```python
from build123d import *

# Parameters (mm, degrees)
SKETCH1_R           = 9.4
BOSS_EXTRUDE1_DEPTH = 13
SKETCH2_R           = 1
BOSS_EXTRUDE2_DEPTH = 5.75
SKETCH3_W           = 7.717079408
SKETCH3_H           = 3.649036098
SKETCH4_R           = 9.4
SKETCH4_R_2         = 0.762
CUT_EXTRUDE1_DEPTH  = 1.617316387


with BuildPart() as part:
    # Sketch1 → Boss-Extrude1 (new body)
    with BuildSketch(Plane.XY):
        with Locations(Location((0, 0, 0), (0, 0, 180))):
            Circle(SKETCH1_R)
    extrude(amount=BOSS_EXTRUDE1_DEPTH)

    # Sketch2 → Boss-Extrude2 (add)
    with BuildSketch(Plane.XY.offset(13)):
        Circle(SKETCH2_R)
    extrude(amount=BOSS_EXTRUDE2_DEPTH)

    # Sketch3 → Cut-Revolve1 (revolve, cut)
    with BuildSketch(Plane(origin=(0, 0, 0), x_dir=(1, 0, 0), z_dir=(0, 1, 0)), mode=Mode.PRIVATE) as cut_revolve1_sk:
        with Locations((5.541460296, -3.441834436)):
            Rectangle(SKETCH3_W, SKETCH3_H)
    revolve(cut_revolve1_sk.sketch.rotate(Axis((0, 0, 0), (0, 0, 1)), 180), axis=Axis((0, 0, 0), (0, 0, 1)), mode=Mode.SUBTRACT)

    # Sketch4 → Cut-Extrude1 (cut)
    with BuildSketch(Plane(origin=(0, 0, 0), x_dir=(-1, 0, 0), z_dir=(0, 0, -1))):
        Circle(SKETCH4_R)
        with BuildLine():
            ThreePointArc((-2.032, 5.588), (0, 7.62), (2.032, 5.588))
            ThreePointArc((2.032, 5.588), (3.073528286, 3.073528286), (5.588, 2.032))
            ThreePointArc((5.588, 2.032), (7.62, 0), (5.588, -2.032))
            ThreePointArc((5.588, -2.032), (3.073528286, -3.073528286), (2.032, -5.588))
            ThreePointArc((2.032, -5.588), (0, -7.62), (-2.032, -5.588))
            ThreePointArc((-2.032, -5.588), (-3.073528286, -3.073528286), (-5.588, -2.032))
            ThreePointArc((-5.588, -2.032), (-7.62, 0), (-5.588, 2.032))
            ThreePointArc((-5.588, 2.032), (-3.073528286, 3.073528286), (-2.032, 5.588))
        make_face(mode=Mode.SUBTRACT)
        with Locations((0, 5.588)):
            Circle(SKETCH4_R_2)
        with Locations((5.588, 0)):
            Circle(SKETCH4_R_2)
        with Locations((0, -5.588)):
            Circle(SKETCH4_R_2)
        with Locations((-5.588, 0)):
            Circle(SKETCH4_R_2)
    extrude(amount=-CUT_EXTRUDE1_DEPTH, mode=Mode.SUBTRACT)


solid = part.part
```
Build history of the part. All positions in model axes, mm. A direction names the side the tool comes from. Round coordinates to 2 decimals unless told otherwise and drop trailing zeros. Order: outer loops, then holes, each group sorted by start corner. A loop starts at its lowest first (then second) coordinate and runs counter-clockwise, first axis right, second up. Notation, with made-up numbers: (3, 6) - (56, 6) arc R8 cw to (56, 15) - close; hole circle Ø10 at (14.5, 82). An arc over 180 degrees is marked (long way). Use a Markdown table: item, result.
1) Tool access for faces 1 (the face through (-2, 0, 1.617)), 2 (the face through (6.35, 0.03, 0.8)), 3 (the face through (3.05, -3.1, 0.8)), 4 (the face through (-7.62, 0.04, 0.8)): list every direction of +Z, -Z, +X, -X, +Y, -Y with a clear straight run to the whole face (end or side of a thin tool).
Recorded:
| item | result |
|---|---|
| face 1 | none |
| face 2 | -Z |
| face 3 | -Z, +X, -Y |
| face 4 | -Z, -X |
2) Saw through at A-A on x = 0. Write the cut outline in (y, z), and give its area (3 significant figures).
Recorded:
| item | result |
|---|---|
| outline | (-9.4, 5.27) - (-1.68, 5.27) - (-1.68, 1.62) - (-4.83, 1.62) - (-4.83, 0) - (4.83, 0) - (4.83, 1.62) - (1.68, 1.62) - (1.68, 5.27) - (9.4, 5.27) - (9.4, 13) - (1, 13) - (1, 18.75) - (-1, 18.75) - (-1, 13) - (-9.4, 13) - close; (-7.62, 0) - (-6.35, 0) - (-6.35, 1.62) - (-7.62, 1.62) - close; (6.35, 0) - (7.62, 0) - (7.62, 1.62) - (6.35, 1.62) - close |
| area | 189 mm² |
3) Flat gauge pins, fed straight in: pin 1 Ø8 at (x, z) = (-6.5, 4.5) entering from -Y; pin 2 Ø0.9 at (x, y) = (0, -5.588) entering from +Z; pin 3 Ø2 at (x, y) = (2.5, -7.5) entering from -Z. Where does each tip first touch, or does it go through?
Recorded:
| item | result |
|---|---|
| pin 1 | stops at y = -9.04 |
| pin 2 | stops at z = 13 |
| pin 3 | stops at z = 5.27 |
4) Pull direction X, two halves, no side cores. Call faces 5 (the face through (0, 0, 0)), 6 (the face through (0.04, 7.62, 0.8)), 7 (the face through (0.17, -6.33, 0.8)), 8 (the face through (0.099, 6.344, 0.797)): pulls with the +X half, pulls with the -X half, needs draft (parallel to the pull), parting line crosses it, or undercut.
Recorded:
| item | result |
|---|---|
| face 5 | needs draft |
| face 6 | parting line crosses it |
| face 7 | undercut |
| face 8 | undercut |
5) Saw through at C-C on y = -4.25. Write the cut outline in (x, z).
Recorded:
| item | result |
|---|---|
| outline | (-8.38, 5.27) - (8.38, 5.27) - (8.38, 13) - (-8.38, 13) - close; (-2.29, 0) - (2.29, 0) - (2.29, 1.62) - (-2.29, 1.62) - close |
6) Wall check: L1, parallel to Y at x = 0, z = 0.8; L2, parallel to Z at x = 4.25, y = -0.5; L3, parallel to Z at x = 0.5, y = 8. Give the ranges that are in metal, low to high.
Recorded:
| item | result |
|---|---|
| L1 | y = -7.62 to -6.35, -4.83 to 4.83, 6.35 to 7.62 |
| L2 | z = 0 to 1.62, 5.27 to 13 |
| L3 | z = 5.27 to 13 |
7) Saw through at D-D on x = -4. Write the cut outline in (y, z).
Recorded:
| item | result |
|---|---|
| outline | (-8.51, 5.27) - (8.51, 5.27) - (8.51, 13) - (-8.51, 13) - close; (-2.41, 0) - (2.41, 0) - (2.41, 1.62) - (-2.41, 1.62) - close |
